The model under review builds one solid part; all positions refer to its coordinate system, in mm. Round coordinates to 2 decimals unless told otherwise and drop trailing zeros. Loops run counter-clockwise (first coordinate to the right, second up) from the corner with the lowest first, then second, coordinate; pieces in that order, holes last. Notation, with made-up numbers: (63, 72.25) -> (90, 72.25) arc R30 cw to (90, 109.25) -> close; hole circle Ø5 at (-18, -2.75). An arc over 180 degrees is marked (long way). Use a Markdown table: item, result. Add a question column.
1) Consider section C-C on z = -13.5. Give the boundary of the cut face in (x, y), plus the area to 3 significant figures.
2) Consider section A-A on z = 0. Give the boundary of the cut face in (x, y).
3) Wall thickness on probe 1 along Z at (x, y) = (31, 1.75); probe 2 along Z at (x, y) = (0, 7.05); probe 3 along Z at (x, y) = (32, 1.5): over which ranges is each line inside the solid? List them lowest first.
4) Consider section D-D on y = 6.5. Give the boundary of the cut face in (x, z).
5) Consider section B-B on x = -31. Give the boundary of the cut face in (y, z), plus the area to 3 significant figures.
6) Insertion check: pin 1 (3 mm diameter, centred on x = 32.5, y = 1, fed in from -Z); pin 2 (1.9 mm diameter, centred on x = 4, z = 13.5, fed in from +Y); pin 3 (4 mm diameter, centred on x = 8.5, y = 3.5, fed in from -Z); pin 4 (8 mm diameter, centred on x = 0, z = 0, fed in from -Y). Each pin has a flat end and moves straight along its axis. Give the tip position at first contact, or say it passes through.
from build123d import *

# Parameters (mm, degrees)
SKETCH_1_R          = 45
EXTRUDE_1_DEPTH     = 4
SKETCH_13_R         = 6
EXTRUDE_5_DEPTH     = 4
SKETCH_15_R         = 1.6
CUT_EXTRUDE_5_DEPTH = 5
CUT_EXTRUDE_6_DEPTH = 5
SKETCH_20_R         = 3.5
CUT_EXTRUDE_7_DEPTH = 5
SKETCH_21_R         = 1.6
CUT_EXTRUDE_8_DEPTH = 5


with BuildPart() as part:
    # Эскиз1 → Бобышка-Вытянуть1 (new body)
    with BuildSketch(Plane(origin=(0, 0, 0), x_dir=(1, 0, 0), z_dir=(0, 1, 0))):
        Circle(SKETCH_1_R)
    extrude(amount=EXTRUDE_1_DEPTH)

    # Эскиз13 → Бобышка-Вытянуть5 (add)
    with BuildSketch(Plane(origin=(0, 4, 0), x_dir=(1, 0, 0), z_dir=(0, 1, 0))):
        Circle(SKETCH_13_R)
    extrude(amount=EXTRUDE_5_DEPTH)

    # Эскиз15 → Вырез-Вытянуть5 (cut, through all)
    with BuildSketch(Plane(origin=(0, 4, 0), x_dir=(1, 0, 0), z_dir=(0, 1, 0))):
        with Locations((-4, 13.5)):
            Circle(SKETCH_15_R)
        with Locations((-4, -13.5)):
            Circle(SKETCH_15_R)
        with Locations((4, -13.5)):
            Circle(SKETCH_15_R)
        with Locations((4, 13.5)):
            Circle(SKETCH_15_R)
    extrude(amount=-CUT_EXTRUDE_5_DEPTH, mode=Mode.SUBTRACT)

    # Эскиз19 → Вырез-Вытянуть6 (cut)
    with BuildSketch(Plane.XZ):
        Polygon((5.05, 2.915618859), (0, 5.831237719), (-5.05, 2.915618859), (-5.05, -2.915618859), (0, -5.831237719), (5.05, -2.915618859), (9.95, -2.915618859), (9.95, 2.915618859), align=None)
    extrude(amount=-CUT_EXTRUDE_6_DEPTH, mode=Mode.SUBTRACT)

    # Эскиз20 → Вырез-Вытянуть7 (cut)
    with BuildSketch(Plane.XZ.offset(-5)):
        Circle(SKETCH_20_R)
    extrude(amount=-CUT_EXTRUDE_7_DEPTH, mode=Mode.SUBTRACT)

    # Эскиз21 → Вырез-Вытянуть8 (cut)
    with BuildSketch(Plane.XZ):
        with Locations((4, 13.5)):
            Circle(SKETCH_21_R)
        with Locations((4, -13.5)):
            Circle(SKETCH_21_R)
        with Locations((31, 13.5)):
            Circle(SKETCH_21_R)
        with Locations((31, -13.5)):
            Circle(SKETCH_21_R)
        with Locations((-31, 13.5)):
            Circle(SKETCH_21_R)
        with Locations((-31, -13.5)):
            Circle(SKETCH_21_R)
    extrude(amount=-CUT_EXTRUDE_8_DEPTH, mode=Mode.SUBTRACT)


solid = part.part
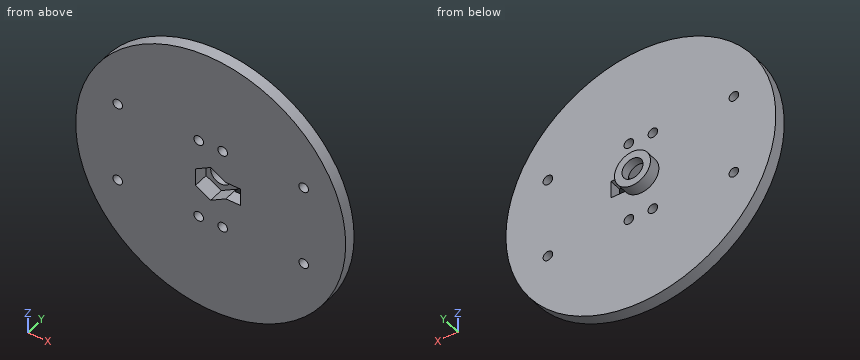
Result set:
| question | item | result |
|---|---|---|
| 1 | outline | (-42.93, 0) -> (-32.6, 0) -> (-32.6, 4) -> (-42.93, 4) -> close; (-29.4, 0) -> (-5.6, 0) -> (-5.6, 4) -> (-29.4, 4) -> close; (-2.4, 0) -> (2.4, 0) -> (2.4, 4) -> (-2.4, 4) -> close; (5.6, 0) -> (29.4, 0) -> (29.4, 4) -> (5.6, 4) -> close; (32.6, 0) -> (42.93, 0) -> (42.93, 4) -> (32.6, 4) -> close |
| 1 | area | 292 mm2 |
| 2 | outline | (-45, 0) -> (-5.05, 0) -> (-5.05, 5) -> (-3.5, 5) -> (-3.5, 8) -> (-6, 8) -> (-6, 4) -> (-45, 4) -> close; (3.5, 5) -> (6, 5) -> (6, 8) -> (3.5, 8) -> close; (9.95, 0) -> (45, 0) -> (45, 4) -> (9.95, 4) -> close |
| 3 | probe 1 | -32.62 to -15.1, -11.9 to 11.9, 15.1 to 32.62 |
| 3 | probe 2 | -6 to -3.5, 3.5 to 6 |
| 3 | probe 3 | -31.64 to -14.75, -12.25 to 12.25, 14.75 to 31.64 |
| 4 | outline | circle Ø12 at (0, 0); hole circle Ø7 at (0, 0) |
| 5 | outline | (0, -32.62) -> (4, -32.62) -> (4, -15.1) -> (0, -15.1) -> close; (0, -11.9) -> (4, -11.9) -> (4, 11.9) -> (0, 11.9) -> close; (0, 15.1) -> (4, 15.1) -> (4, 32.62) -> (0, 32.62) -> close |
| 5 | area | 235 mm2 |
| 6 | pin 1 | z = -32.62 |
| 6 | pin 2 | through |
| 6 | pin 3 | z = -44.53 |
| 6 | pin 4 | y = 5 |
